from build123d import *

# Parameters (mm, degrees)
BOSS_EXTRUDE1_DEPTH      = 72.1
BOSS_EXTRUDE1_DEPTH_BACK = 72.1
SKETCH1_R                = 30
BOSS_EXTRUDE2_DEPTH      = 36.05
BOSS_EXTRUDE3_DEPTH      = 36.05
BOSS_EXTRUDE3_DEPTH_BACK = 36.05
SKETCH5_R                = 9
CUT_EXTRUDE1_DEPTH       = 8
FILLET1_R                = 5


with BuildPart() as part:
    # Sketch1 → Boss-Extrude1 (new, two sides: drawn at the far end of the back side and taken through both)
    with BuildSketch(Plane(origin=(0, 0, 0), x_dir=(0, 0, -1), z_dir=(1, 0, 0)).offset(-BOSS_EXTRUDE1_DEPTH_BACK)):
        Circle(SKETCH1_R)
    extrude(amount=BOSS_EXTRUDE1_DEPTH + BOSS_EXTRUDE1_DEPTH_BACK)

    # Sketch3 → Boss-Extrude2 (add)
    with BuildSketch(Plane(origin=(72.1, 0, 0), x_dir=(0, 0, -1), z_dir=(1, 0, 0))):
        with BuildLine():
            Line((7.607128711, 16.313540167), (21.130913087, 45.315389352))
            ThreePointArc((21.130913087, 45.315389352), (0, 50), (-21.130913087, 45.315389352))
            Line((-21.130913087, 45.315389352), (-7.607128711, 16.313540167))
            ThreePointArc((-7.607128711, 16.313540167), (0, 18), (7.607128711, 16.313540167))
        make_face()
    extrude(amount=-BOSS_EXTRUDE2_DEPTH)

    # Mirror1: part across plane


with BuildPart() as part_1:
    add(part.part)
    add(part.part.mirror(Plane(origin=(0, 0, 0), x_dir=(0, 0, 1), z_dir=(1, 0, 0))))

    # Sketch4 → Boss-Extrude3 (add, two sides: drawn at the far end of the back side and taken through both)
    with BuildSketch(Plane(origin=(0, 0, 0), x_dir=(0, 0, -1), z_dir=(1, 0, 0)).offset(-BOSS_EXTRUDE3_DEPTH_BACK)):
        with BuildLine():
            Line((-7.607128711, -16.313540167), (-21.130913087, -45.315389352))
            ThreePointArc((-21.130913087, -45.315389352), (0, -50), (21.130913087, -45.315389352))
            Line((21.130913087, -45.315389352), (7.607128711, -16.313540167))
            ThreePointArc((7.607128711, -16.313540167), (0, -18), (-7.607128711, -16.313540167))
        make_face()
    extrude(amount=BOSS_EXTRUDE3_DEPTH + BOSS_EXTRUDE3_DEPTH_BACK)

    # Sketch5 → Cut-Extrude1 (cut)
    with BuildSketch(Plane(origin=(72.1, 0, 0), x_dir=(0, 0, -1), z_dir=(1, 0, 0))):
        Circle(SKETCH5_R)
    cut_extrude1 = extrude(amount=-CUT_EXTRUDE1_DEPTH, mode=Mode.SUBTRACT)

    # Mirror3: Cut-Extrude1 across plane
    add(cut_extrude1.mirror(Plane(origin=(0, 0, 0), x_dir=(0, 0, 1), z_dir=(1, 0, 0))), mode=Mode.SUBTRACT)

    # Fillet1
    fillet1_edges = [part_1.edges().sort_by_distance(p)[0] for p in [
        (54.075, 27.189233611, 12.678547852),
        (54.075, 27.189233611, -12.678547852),
        (-54.075, 27.189233611, 12.678547852),
        (-54.075, 27.189233611, -12.678547852),
        (0, -27.189233611, -12.678547852),
        (0, -27.189233611, 12.678547852),
    ]]
    fillet(fillet1_edges, radius=FILLET1_R)


solid = part_1.part
The model under review builds one solid part; all positions refer to its coordinate system, in mm. A direction names the side the tool comes from. Round coordinates to 2 decimals unless told otherwise and drop trailing zeros. Loops run counter-clockwise (first coordinate to the right, second up) from the corner with the lowest first, then second, coordinate; pieces in that order, holes last. Notation, with made-up numbers: (-30.5, -9.5) - (2.5, -9.5) arc R30 cw to (2.5, 24.5) - close; hole circle Ø3 at (86.25, 20). An arc over 180 degrees is marked (long way). Use CSV: the item, a comma, the result in double quotes.
(1) Machinability: for faces 4 (the flat face through (-0.5, -38.45, -17.93)), 5 (the cylindrical face through (-68.156, 8.923, 1.172)), 6 (the flat face through (64.1, 0, 0)), which of the approach directions +Z, -Z, +X, -X, +Y, -Y give a long, thin tool a straight path to every point of the face, cutting with its end or side? Answer none if there is none.
Working result:
face 4,"-Z, +X, -X"
face 5,"-X"
face 6,"+X"
(2) Clearance check with flat-ended pins moving along their axes: P1, Ø10, axis at x = 2, z = 6, coming from the +Y side; P2, Ø12, axis at y = -37, z = -4.5, coming from the +X side; P3, Ø11, axis at y = 0, z = 0, coming from the +X side; P4, Ø20, axis at y = -2, z = -4, coming from the +X side. State where each tip first meets the part, or that it passes through.
Working result:
P1,"stops at y = 29.98"
P2,"stops at x = 36.05"
P3,"stops at x = 64.1"
P4,"stops at x = 72.1"
(3) Take a section at A-A, the plane z = 0. Give the boundary of the cut face in (x, y).
Working result:
outline,"(-72.1, -30) - (-36.05, -30) - (-36.05, -50) - (36.05, -50) - (36.05, -30) - (72.1, -30) - (72.1, -9) - (64.1, -9) - (64.1, 9) - (72.1, 9) - (72.1, 50) - (36.05, 50) - (36.05, 30) - (-36.05, 30) - (-36.05, 50) - (-72.1, 50) - (-72.1, 9) - (-64.1, 9) - (-64.1, -9) - (-72.1, -9) - close"
(4) Take a section at D-D, the plane y = 27. Give the boundary of the cut face in (x, z).
Working result:
outline,"(-72.1, -14.72) - (-36.05, -14.72) - (-36.05, -13.08) - (36.05, -13.08) - (36.05, -14.72) - (72.1, -14.72) - (72.1, 14.72) - (36.05, 14.72) - (36.05, 13.08) - (-36.05, 13.08) - (-36.05, 14.72) - (-72.1, 14.72) - close"
(5) For line 1 (Y direction, x = -66.5, z = 0); line 2 (X direction, y = 46, z = -2); line 3 (Y direction, x = 20, z = 15.5), list the stretches that pass through material, from the lowest coordinate up.
Working result:
line 1,"y = -30 to -9, 9 to 50"
line 2,"x = -72.1 to -36.05, 36.05 to 72.1"
line 3,"y = -47.54 to -33.24, -25.89 to 25.69"
(6) Take a section at B-B, the plane y = 0. Give the boundary of the cut face in (x, z).
Working result:
outline,"(-72.1, -30) - (72.1, -30) - (72.1, -9) - (64.1, -9) - (64.1, 9) - (72.1, 9) - (72.1, 30) - (-72.1, 30) - (-72.1, 9) - (-64.1, 9) - (-64.1, -9) - (-72.1, -9) - close"
(7) Take a section at C-C, the plane x = -27.5. Give the boundary of the cut face in (y, z).
Working result:
outline,"(-45.32, -21.13) - (-31.4, -14.64) arc R5 cw to (-25.1, -16.43) arc R30 ccw (long way) to (-25.1, 16.43) arc R5 cw to (-31.4, 14.64) - (-45.32, 21.13) arc R50 ccw to start"
(8) The part is to be moulded in two halves that separate along Y. For faces 1 (the cylindrical face through (-54, 50, 0)), 2 (the flat face through (-0.5, -38.26, 17.84)), 3 (the flat face through (-72.1, 11, 0)), say which applies: pulls with the +Y half, pulls with the -Y half, needs draft (parallel to the pull), parting line crosses it, or undercut.
Working result:
face 1,"pulls with the +Y half"
face 2,"undercut"
face 3,"needs draft"
